Can you work these out from the drawing? Everything is in mm from the part's minimum corner. Give positions to 0.01 mm unless a question says otherwise; leave off trailing zeros. Loops run counter-clockwise (first coordinate to the right, second up) from the corner with the lowest first, then second, coordinate; pieces in that order, holes last. Notation, with made-up numbers: (-14, 48) - (40, 48) arc R31 ccw to (40, 73) - close; hole circle Ø8 at (22, 15). An arc over 180 degrees is marked (long way). One line per item, written item: value. Start each with the question number.
Q1. I want a section at C-C (y = 6.35). Please give me the cut outline in (x, z), then the cut area to 3 significant figures.
Q2. If I drill on line 1 (X direction, y = 5.5, z = 6.35); line 2 (X direction, y = 6.35, z = 9); line 3 (X direction, y = 6.35, z = 4.25), over which ranges is the centre line in solid material (lowest first)? Write a range as from..to.
Q3. I want a section at D-D (x = 41.5). Please give me the cut outline in (y, z).
Q4. I'm going to push a flat-ended pin straight in: P1, Ø1.5, axis at x = 46.5, z = 10, coming from the -Y side. Where does the tip first touch, or does it pass through?
Q5. If we mould it in two halves opening along X, with no side actions, what happens to the marked faces 1, 2 and 3? For each: released by +X, released by -X, zero draft, split by the parting line, or undercut.
Q6. I want a section at A-A (x = 5). Please give me the cut outline in (y, z), then the cut area to 3 significant figures.
Q7. I want a section at B-B (z = 6.5). Please give me the cut outline in (x, y).
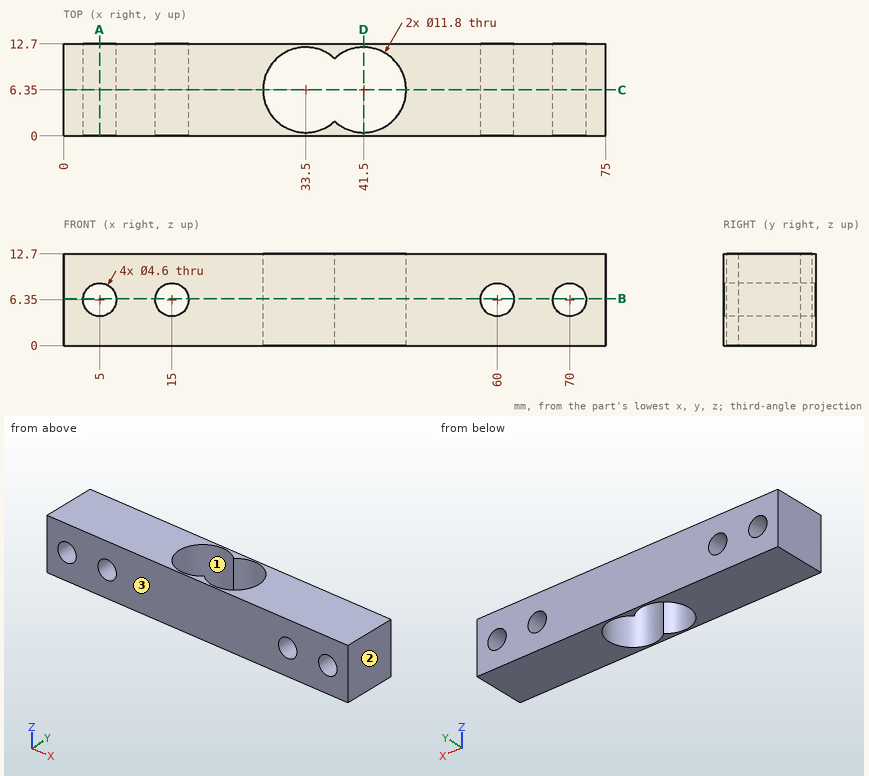
Worked answers:
1. outline: (0, 0) - (27.6, 0) - (27.6, 12.7) - (0, 12.7) - close; (47.4, 0) - (75, 0) - (75, 12.7) - (47.4, 12.7) - close; hole circle Ø4.6 at (5, 6.35); hole circle Ø4.6 at (15, 6.35); hole circle Ø4.6 at (60, 6.35); hole circle Ø4.6 at (70, 6.35)
1. area: 635 mm²
2. line 1: x = 0..2.7, 7.3..12.7, 17.3..27.66, 47.34..57.7, 62.3..67.7, 72.3..75
2. line 2: x = 0..27.6, 47.4..75
2. line 3: x = 0..4.06, 5.94..14.06, 15.94..27.6, 47.4..59.06, 60.94..69.06, 70.94..75
3. outline: (0, 0) - (0.45, 0) - (0.45, 12.7) - (0, 12.7) - close; (12.25, 0) - (12.7, 0) - (12.7, 12.7) - (12.25, 12.7) - close
4. P1: stops at y = 0
5. face 1: undercut
5. face 2: released by +X
5. face 3: zero draft
6. outline: (0, 0) - (12.7, 0) - (12.7, 4.05) - (0, 4.05) - close; (0, 8.65) - (12.7, 8.65) - (12.7, 12.7) - (0, 12.7) - close
6. area: 103 mm²
7. outline: (0, 0) - (2.7, 0) - (2.7, 12.7) - (0, 12.7) - close; (7.3, 0) - (12.7, 0) - (12.7, 12.7) - (7.3, 12.7) - close; (17.3, 0) - (57.7, 0) - (57.7, 12.7) - (17.3, 12.7) - close; (62.3, 0) - (67.7, 0) - (67.7, 12.7) - (62.3, 12.7) - close; (72.3, 0) - (75, 0) - (75, 12.7) - (72.3, 12.7) - close; hole (37.5, 2.01) arc R5.9 ccw (long way) to (37.5, 10.69) arc R5.9 ccw (long way) to start
